```python
from build123d import *

# Parameters (mm, degrees)
SKETCH1_R           = 2.75
BOSS_EXTRUDE1_DEPTH = 7
SKETCH2_R           = 2.35
CUT_EXTRUDE1_DEPTH  = 23.737634002
SKETCH3_R           = 5.25
CUT_EXTRUDE2_DEPTH  = 5
CHAMFER1_SIZE       = 0.5
SKETCH4_R           = 4.5
CUT_EXTRUDE3_DEPTH  = 6


with BuildPart() as part:
    # Sketch1 → Boss-Extrude1 (new, symmetric)
    with BuildSketch(Plane.XY):
        with BuildLine():
            Line((12, -6), (-12, -6))
            ThreePointArc((-12, -6), (-18, 0), (-12, 6))
            Line((-12, 6), (12, 6))
            ThreePointArc((12, 6), (18, 0), (12, -6))
        make_face()
        with Locations((-12, 0)):
            Circle(SKETCH1_R, mode=Mode.SUBTRACT)
        with Locations((12, 0)):
            Circle(SKETCH1_R, mode=Mode.SUBTRACT)
    extrude(amount=BOSS_EXTRUDE1_DEPTH, both=True)

    # Sketch2 → Cut-Extrude1 (cut, through all)
    with BuildSketch(Plane(origin=(0, 6, 0), x_dir=(1, 0, 0), z_dir=(0, 1, 0))):
        with Locations(Location((0, 0, 0), (0, 0, 180))):
            Circle(SKETCH2_R)
    extrude(amount=-CUT_EXTRUDE1_DEPTH, mode=Mode.SUBTRACT)

    # Sketch3 → Cut-Extrude2 (cut)
    with BuildSketch(Plane(origin=(0, 6, 0), x_dir=(1, 0, 0), z_dir=(0, 1, 0))):
        with Locations(Location((0, 0, 0), (0, 0, 180))):
            Circle(SKETCH3_R)
    extrude(amount=-CUT_EXTRUDE2_DEPTH, mode=Mode.SUBTRACT)

    # Chamfer1
    chamfer1_edges = [part.edges().sort_by_distance(p)[0] for p in [
        (-18, 0, 7),
        (0, -6, 7),
        (18, 0, 7),
        (0, 6, 7),
    ]]
    chamfer(chamfer1_edges, length=CHAMFER1_SIZE)

    # Sketch4 → Cut-Extrude3 (cut)
    with BuildSketch(Plane.XY.offset(7)):
        with Locations((-12, 0)):
            Circle(SKETCH4_R)
        with Locations((12, 0)):
            Circle(SKETCH4_R)
    extrude(amount=-CUT_EXTRUDE3_DEPTH, mode=Mode.SUBTRACT)


solid = part.part
```
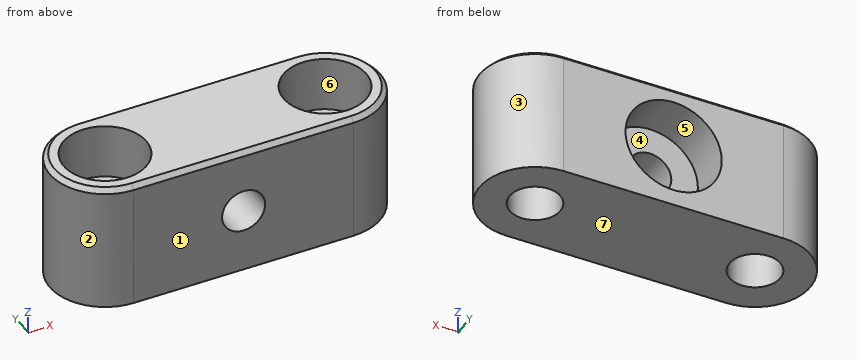
Can you work these out from the model? Positions are in its coordinate system, mm. Face numbers are marked on the shaded views. A direction names the side the tool comes from. Coordinates: 2 decimals unless noted, no trailing zeros. Loops run counter-clockwise (first coordinate to the right, second up) from the corner with the lowest first, then second, coordinate; pieces in that order, holes last. Notation, with made-up numbers: M -29.75,43.5 L -5.75,43.5 A31 ccw -5.75,68.5 Z; hole C 76,71.5 d3. An arc over 180 degrees is marked long. Put each result on its own line as item: value. Start each with the question number.
(1) Imagine slicing it at D-D on z = -1.75. List the corners of the cut face in (x, y) for me, and give its area (3 significant figures).
(2) Imagine slicing it at B-B on z = 0. List the corners of the cut face in (x, y) for me, and give its area (3 significant figures).
(3) I need wall thicknesses on probe 1 along X at (y, z) = (0, -4.25); probe 2 along Y at (x, z) = (12, 3.1); probe 3 along X at (y, z) = (0.5, 2). Which ranges of each line are inside material? Lowest first, please.
(4) We'd pull the mould along X, two halves only. Please class the marked faces 1, 2, 3 and 4: +X half, -X half, draft (parallel to the pull), parting line (faces both ways), or undercut.
(5) Imagine slicing it at C-C on x = 0. List the corners of the cut face in (y, z) for me.
(6) Which directions (+Z, -Z, +X, -X, +Y, -Y) give clear straight access to the entire face, cutting with the end or side of a thin tool? Please do the marked faces 5, 6 and 7.
(7) Will this pin go through, and if not, where does the flat tip stop? pin 1 Ø6.5 at (x, y) = (-12, 0) entering from +Z.
(8) Imagine slicing it at A-A on y = 0. List the corners of the cut face in (x, z) for me.
Worked answers:
1. outline: M -12,-6 L -1.57,-6 L -1.57,1 L -4.95,1 L -4.95,6 L -12,6 A6 ccw Z; M 1.57,-6 L 12,-6 A6 ccw 12,6 L 4.95,6 L 4.95,1 L 1.57,1 Z; hole C -12,0 d5.5; hole C 12,0 d5.5
1. area: 282 mm2
2. outline: M -12,-6 L -2.35,-6 L -2.35,1 L -5.25,1 L -5.25,6 L -12,6 A6 ccw Z; M 2.35,-6 L 12,-6 A6 ccw 12,6 L 5.25,6 L 5.25,1 L 2.35,1 Z; hole C -12,0 d5.5; hole C 12,0 d5.5
2. area: 268 mm2
3. probe 1: x = -18 to -14.75, -9.25 to 9.25, 14.75 to 18
3. probe 2: y = -6 to -4.5, 4.5 to 6
3. probe 3: x = -17.98 to -16.47, -7.53 to -1.23, 1.23 to 7.53, 16.47 to 17.98
4. face 1: draft
4. face 2: -X half
4. face 3: +X half
4. face 4: undercut
5. outline: M -6,-7 L 6,-7 L 6,-5.25 L 1,-5.25 L 1,-2.35 L -6,-2.35 Z; M -6,2.35 L 1,2.35 L 1,5.25 L 6,5.25 L 6,6.5 L 5.5,7 L -5.5,7 L -6,6.5 Z
6. face 5: +Y
6. face 6: +Z
6. face 7: -Z, +X, -X, +Y, -Y
7. pin 1: stops at z = 1
8. outline: M -18,-7 L -14.75,-7 L -14.75,1 L -16.5,1 L -16.5,7 L -17.5,7 L -18,6.5 Z; M -9.25,-7 L 9.25,-7 L 9.25,1 L 7.5,1 L 7.5,7 L -7.5,7 L -7.5,1 L -9.25,1 Z; M 14.75,-7 L 18,-7 L 18,6.5 L 17.5,7 L 16.5,7 L 16.5,1 L 14.75,1 Z; hole C 0,0 d4.7
